For this review, take the finished solid that the model builds, in its own axes (mm). Give positions to 0.01 mm unless a question says otherwise; leave off trailing zeros. Write each loop counter-clockwise with the first axis right and the second up, starting at its lowest first coordinate (ties: lowest second). Pieces come first, ordered by that corner, then holes. Notation, with made-up numbers: (-9, 31.5) -> (13, 31.5) arc R8 cw to (13, 42.5) -> close; hole circle Ø5 at (-16.75, -20.5). An arc over 180 degrees is marked (long way). Answer as CSV lines item,"result".
```python
from build123d import *

# Parameters (mm, degrees)
EXTRUDE_1_OUTLINE_R      = 50
EXTRUDE_1_OUTLINE_R_2    = 47
EXTRUDE_1_DEPTH          = 200
CUT_EXTRUDE_1_DEPTH      = 213.132034356
CUT_EXTRUDE_1_DEPTH_BACK = 213.132034356
SKETCH_2_R               = 66.5


# Read off the part's stored shape, not the designer's step: Вытянуть-Тонкостенный1
with BuildPart() as part:
    # Вытянуть-Тонкостенный1 outline → Вытянуть-Тонкостенный1 (new body)
    with BuildSketch(Plane(origin=(0, 0, 0), x_dir=(1, 0, 0), z_dir=(0, 1, 0))):
        Circle(EXTRUDE_1_OUTLINE_R)
        Circle(EXTRUDE_1_OUTLINE_R_2, mode=Mode.SUBTRACT)
    extrude(amount=EXTRUDE_1_DEPTH)

    # Эскиз2 → Вырез-Вытянуть1 (cut, two sides: drawn at the far end of the back side and taken through both)
    with BuildSketch(Plane(origin=(0, 0, 0), x_dir=(1, 0, 0), z_dir=(0, -0.5735764363510444, -0.819152044288993)).offset(-CUT_EXTRUDE_1_DEPTH_BACK)):
        with Locations((0, -180)):
            Circle(SKETCH_2_R)
    extrude(amount=CUT_EXTRUDE_1_DEPTH + CUT_EXTRUDE_1_DEPTH_BACK, mode=Mode.SUBTRACT)


solid = part.part
```
Q1. Add section B-B (y = 78). Write out the cut boundary in (x, z).
Answer block:
outline,"circle Ø100 at (0, 0); hole circle Ø94 at (0, 0)"
Q2. To check wall thickness, follow probe 1 along Z at (x, y) = (0, 65); probe 2 along X at (y, z) = (131, -15). State the ranges of each line that lie inside material, in increasing order. Write a range as [from, to].
Answer block:
probe 1,"z = [-50, -47], [47, 50]"
probe 2,"x = [-47.7, -44.54], [44.54, 47.7]"
Q3. Add section A-A (x = -36). Write out the cut boundary in (y, z).
Answer block:
outline,"(0, -34.7) -> (127.19, -34.7) -> (130.33, -30.22) -> (0, -30.22) -> close; (0, 30.22) -> (172.64, 30.22) -> (175.78, 34.7) -> (0, 34.7) -> close"
Q4. Add section C-C (x = 0). Write out the cut boundary in (y, z), plus the area to 3 significant figures.
Answer block:
outline,"(0, -50) -> (103.55, -50) -> (105.65, -47) -> (0, -47) -> close; (0, 47) -> (171.47, 47) -> (173.57, 50) -> (0, 50) -> close"
area,"831 mm2"
Q5. Clearance check with flat-ended pins moving along their axes: pin 1 (3 mm diameter, centred on x = -5, y = 53.5, fed in from -Z); pin 2 (1.5 mm diameter, centred on x = -1, y = 62.5, fed in from +Z); pin 3 (3 mm diameter, centred on y = 45.5, z = -23, fed in from +X). State where each tip first meets the part, or that it passes through.
Answer block:
pin 1,"stops at z = -49.88"
pin 2,"stops at z = 50"
pin 3,"stops at x = 45.14"
Q6. Draft analysis for pull direction X (two halves, no side actions). For faces 1 (the cylindrical face through (-10.84, 86.73, 48.81)), 2 (the cylindrical face through (-10.189, 85.173, 45.882)), 3 (the flat face through (-34, 0, 33)), state which applies: released by +X, released by -X, zero draft, split by the parting line, or undercut.
Answer block:
face 1,"split by the parting line"
face 2,"undercut"
face 3,"zero draft"
